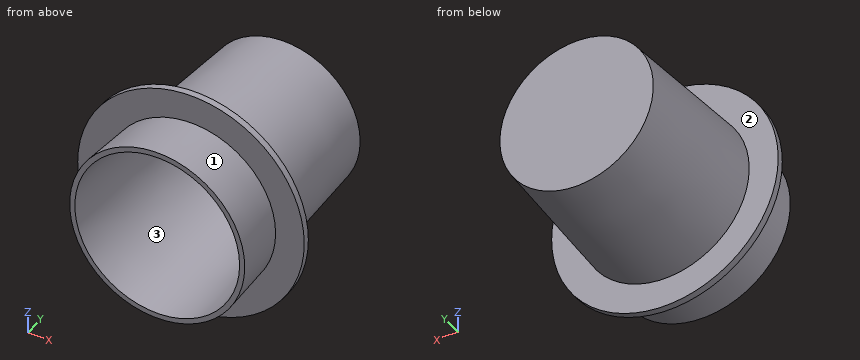
```python
from build123d import *

# Parameters (mm, degrees)
F0_R     = 107.95
F1_DEPTH = 254
F1_TAPER = 3
F2_R     = 101.6
F3_DEPTH = 241.3
F3_TAPER = 3
F6_R     = 139.7
F6_R_2   = 103.9495
F7_DEPTH = 8.255


with BuildPart() as f1:
    # F0 (on Front) → F1 (new body)
    with BuildSketch(Plane.XZ):
        Circle(F0_R)
    extrude(amount=-F1_DEPTH, taper=F1_TAPER)

    # F2 (on face) → F3 (cut)
    with BuildSketch(Plane.XZ):
        Circle(F2_R)
    extrude(amount=-F3_DEPTH, taper=F3_TAPER, mode=Mode.SUBTRACT)

    # F6 (on offset) → F7 (join)
    with BuildSketch(Plane.XZ.offset(-76.2)):
        Circle(F6_R)
        Circle(F6_R_2, mode=Mode.SUBTRACT)
    extrude(amount=F7_DEPTH)


solid = f1.part
```
Read the model definition and answer for the solid it produces. Units are mm, in the model's axes. Face numbers are marked on the shaded views. Coordinates: 2 decimals unless noted, no trailing zeros. Write each loop counter-clockwise with the first axis right and the second up, starting at its lowest first coordinate (ties: lowest second). Pieces come first, ordered by that corner, then holes. Notation, with made-up numbers: (-14.75, 84.25) - (17.25, 84.25) arc R13 ccw to (17.25, 90.25) - close; hole circle Ø11 at (85.5, 19). An arc over 180 degrees is marked (long way). Answer as a JSON object with one key per item and string values. Group by question number.
1. The mould has two halves that part along Y. Classify the marked faces 1, 2 and 3: +Y half, -Y half, draft (parallel to the pull), parting line (faces both ways), or undercut.
2. A cutting plane is placed at C-C (y = 204). Determine the outline of the cut face in (x, z), plus the area to 3 significant figures.
3. Consider L1, parallel to Y at x = 77, z = -14.5; L2, parallel to Y at x = -104, z = 65 (3 decimals); L3, parallel to X at y = 103, z = -35. Determine where each line is inside the solid, lowest interval first. Write a range as [from, to].
4. A cutting plane is placed at A-A (x = 0). Determine the outline of the cut face in (y, z) (3 decimals).
5. A cutting plane is placed at B-B (y = 18). Determine the outline of the cut face in (x, z).
6. Each of these flat-tipped pins is pushed along its axis until it touches: P1, Ø1, axis at x = -47, z = 100, coming from the +Y side; P2, Ø12, axis at x = -60.5, y = 77.5, coming from the +Z side; P3, Ø6, axis at y = 219.5, z = 33.5, coming from the +X side. Where does it stop, or does it pass through?
Worked out:
{
 "1": {"face 1": "undercut", "face 2": "+Y half", "face 3": "-Y half"},
 "2": {"outline": "circle Ø194.52 at (0, 0); hole circle Ø181.82 at (0, 0)", "area": "3,750 mm²"},
 "3": {"L1": "y = [241.3, 254]", "L2": "y = [67.945, 76.2]", "L3": "x = [-96.39, -89.61], [89.61, 96.39]"},
 "4": {"outline": "(0, -107.95) - (67.945, -104.389) - (67.945, -139.7) - (76.2, -139.7) - (76.2, -103.957) - (254, -94.638) - (254, 94.638) - (76.2, 103.957) - (76.2, 139.7) - (67.945, 139.7) - (67.945, 104.389) - (0, 107.95) - (0, 101.6) - (241.3, 88.954) - (241.3, -88.954) - (0, -101.6) - close"},
 "5": {"outline": "circle Ø214.01 at (0, 0); hole circle Ø201.31 at (0, 0)"},
 "6": {"P1": "stops at y = 76.2", "P2": "stops at z = 128.57", "P3": "stops at x = 91.51"}
}
